```python
from build123d import *

# Parameters (mm, degrees)
SKETCH1_R              = 3.175
BOSS_EXTRUDE1_DEPTH    = 79.375
ATTACHHMENT_HOLE_D     = 3.7973
ATTACHHMENT_HOLE_DEPTH = 12.7
ATTACHHMENT_HOLE_TIP   = 1.140824014
F_10_24_TAPPED_D       = 3.7973
F_10_24_TAPPED_DEPTH   = 12.7
F_10_24_TAPPED_TIP     = 1.140824014


with BuildPart() as part:
    # Sketch1 → Boss-Extrude1 (new body)
    with BuildSketch(Plane(origin=(0, 0, 0), x_dir=(1, 0, 0), z_dir=(0, 1, 0))):
        with Locations(Location((0, 0, 0), (0, 0, 90))):
            Circle(SKETCH1_R)
    extrude(amount=BOSS_EXTRUDE1_DEPTH)

    # Attachhment Hole
    with Locations(Plane(origin=(0, 79.375, 0), x_dir=(1, 0, 0), z_dir=(0, 1, 0))):
        with Locations((0, 0)):
            Hole(ATTACHHMENT_HOLE_D / 2, depth=ATTACHHMENT_HOLE_DEPTH)
            with Locations((0, 0, -(ATTACHHMENT_HOLE_DEPTH + ATTACHHMENT_HOLE_TIP / 2))):  # 118° drill point
                Cone(0, ATTACHHMENT_HOLE_D / 2, ATTACHHMENT_HOLE_TIP, mode=Mode.SUBTRACT)

    # #10-24 Tapped
    with Locations(Plane(origin=(0, 0, 0), x_dir=(-1, 0, 0), z_dir=(0, -1, 0))):
        with Locations((0, 0)):
            Hole(F_10_24_TAPPED_D / 2, depth=F_10_24_TAPPED_DEPTH)
            with Locations((0, 0, -(F_10_24_TAPPED_DEPTH + F_10_24_TAPPED_TIP / 2))):  # 118° drill point
                Cone(0, F_10_24_TAPPED_D / 2, F_10_24_TAPPED_TIP, mode=Mode.SUBTRACT)


solid = part.part
```
For this review, take the finished solid that the model builds, in its own axes (mm). A direction names the side the tool comes from. Round coordinates to 2 decimals unless told otherwise and drop trailing zeros. Write each loop counter-clockwise with the first axis right and the second up, starting at its lowest first coordinate (ties: lowest second). Pieces come first, ordered by that corner, then holes. Notation, with made-up numbers: M 22,85.5 L 48,85.5 A27 ccw 48,102.5 Z; hole C -32,15.5 d10. An arc over 180 degrees is marked long. One line per item, written item: value. Start each with the question number.
(1) We need section B-B (y = 20). Give the boundary of the cut face in (x, z) (3 decimals), and give its area (3 significant figures).
(2) We need section A-A (y = 7.5). Give the boundary of the cut face in (x, z) (3 decimals), and give its area (3 significant figures).
(3) Wall thickness on line 1 (X direction, y = 11.5, z = -0.25); line 2 (Z direction, x = -0.75, y = 71): over which ranges is each line inside the solid? List them lowest first.
(4) The part is to be moulded in two halves that separate along Z. For faces 1 (the flat face through (2.1, 0, 0)), 2 (the cylindrical face through (1.93, 39.13, 2.52)), 3 (the conical face through (0.31, 65.73, -0.1)), 4 (the cylindrical face through (1.8, 6.4, -0.6)), say which applies: released by +Z, released by -Z, zero draft, split by the parting line, or undercut.
(5) Machinability: for faces 5 (the flat face through (2.1, 79.375, 0)), 6 (the cylindrical face through (-1.8, 72.9, -0.6)), which of the approach directions +Z, -Z, +X, -X, +Y, -Y give a long, thin tool a straight path to every point of the face, cutting with its end or side? Answer none if there is none.
(6) Insertion check: pin 1 (2 mm diameter, centred on y = 17.5, z = 2.5, fed in from -X); pin 2 (2.5 mm diameter, centred on x = 0, z = 0, fed in from +Y). Each pin has a flat end and moves straight along its axis. Give the tip position at first contact, or say it passes through.
Result:
1. outline: C 0,0 d6.35
1. area: 31.7 mm²
2. outline: C 0,0 d6.35; hole C 0,0 d3.797
2. area: 20.3 mm²
3. line 1: -3.17 to -1.88, 1.88 to 3.17
3. line 2: -3.09 to -1.74, 1.74 to 3.09
4. face 1: zero draft
4. face 2: split by the parting line
4. face 3: undercut
4. face 4: undercut
5. face 5: +Z, -Z, +X, -X, +Y
5. face 6: +Y
6. pin 1: x = -2.8
6. pin 2: y = 66.29
